Source: CAD feature listing. Evaluate the final solid. Frame: model axes, mm. Face numbers are marked on the shaded views. A direction names the side the tool comes from. Give positions to 0.01 mm unless a question says otherwise; leave off trailing zeros. Order: outer loops, then holes, each group sorted by start corner. A loop starts at its lowest first (then second) coordinate and runs counter-clockwise, first axis right, second up. Notation, with made-up numbers: (54, -5) - (67, -5) arc R18 cw to (67, 19) - close; hole circle Ø6 at (41.25, 1). An arc over 180 degrees is marked (long way). Answer as CSV lines item,"result".
Autodesk Inventor part; units mm, degrees
ref_plane "YZ Plane" through (0, 0, 0) normal (1, 0, 0) x (0, 1, 0)
ref_plane "XZ Plane" through (0, 0, 0) normal (0, 1, 0) x (-1, 0, 0)
ref_plane "XY Plane" through (0, 0, 0) normal (0, 0, 1) x (1, 0, 0)
sketch "Sketch2" plane through (0, 0, 0) normal (0, 1, 0) x (-1, 0, 0)
  circle A0 centre (0, 0) radius 21
  dimension "d1" = 42
extrude "Extrusion1" add sketch "Sketch2" along normal mid plane 16
sketch "Sketch3" plane through (0, -8, 0) normal (0, -1, 0) x (1, 0, 0)
  circle A0 centre (0, 0) radius 21
  dimension "d4" = 42
ref_plane "Work Plane1" through (0, -38, 0) normal (0, -1, 0) x (1, 0, 0)
sketch "Sketch4" plane through (0, -38, 0) normal (0, -1, 0) x (1, 0, 0)
  circle A0 centre (0, 0) radius 28.77
  dimension "d6" = 57.54
loft "Loft1" add profiles "Sketch4" section 1 edges at (21, -8, 0)
sketch "Sketch5" plane through (0, -38, 0) normal (0, -1, 0) x (1, 0, 0)
  circle A0 centre (0, 0) radius 28.77
  line L0 (0, 0) -> (28.77, 0) construction
  line L1 (0, 36.3025) -> (31.4389, 18.1512)
  line L2 (31.4389, 18.1512) -> (31.4389, -18.1512)
  line L3 (31.4389, -18.1512) -> (0, -36.3025)
  line L4 (0, -36.3025) -> (-31.4389, -18.1512)
  line L5 (-31.4389, -18.1512) -> (-31.4389, 18.1512)
  line L6 (-31.4389, 18.1512) -> (0, 36.3025)
ref_plane "Work Plane2" through (0, -68, 0) normal (0, -1, 0) x (1, 0, 0)
sketch "Sketch6" plane through (0, -38, 0) normal (0, -1, 0) x (1, 0, 0)
  point P0 (0, 0)
sketch "Sketch8" plane through (0, -68, 0) normal (0, -1, 0) x (1, 0, 0)
  line L0 (0, 47.0378) -> (40.7359, 23.5189)
  line L1 (40.7359, 23.5189) -> (40.7359, -23.5189)
  line L2 (40.7359, -23.5189) -> (0, -47.0378)
  line L3 (0, -47.0378) -> (-40.7359, -23.5189)
  line L4 (-40.7359, -23.5189) -> (-40.7359, 23.5189)
  line L5 (-40.7359, 23.5189) -> (0, 47.0378)
  point P0 (0, 0)
  point P1 (0, 0)
loft "Loft3" add profiles "Sketch8", "Sketch5" contours all / A0 | L1 L2 L3 L4 L5 L6
sketch "Sketch9" plane through (-40.7359, -68, -23.5189) normal (-0.9551836, 0.296014, 0) x (0, 0, 1)
  line L0 (0, 0) -> (47.0378, 0)
  line L1 (23.5189, 0) -> (16.0189, 0)
  line L2 (31.0189, 0) -> (23.5189, 0)
  line L3 (31.0189, 0) -> (16.0189, 0)
  line L4 (16.0189, 20) -> (31.0189, 20)
  line L5 (23.5189, 0) -> (8.5189, 0)
  line L6 (8.5189, 0) -> (8.5189, 20)
  line L7 (8.5189, 20) -> (38.5189, 20)
  line L8 (38.5189, 20) -> (38.5189, 0)
  point P0 (23.5189, 77.0109)
  dimension "d40" = 15
  dimension "d41" = 20
  dimension "d42" = 30
sketch "Sketch10" plane through (40.7359, -68, 23.5189) normal (0.9551836, 0.296014, 0) x (0, 0, -1)
  line L0 (38.5189, 20) -> (38.5189, 0)
  line L1 (8.5189, 0) -> (8.5189, 20)
  line L2 (8.5189, 20) -> (38.5189, 20)
  line L3 (38.5189, 20) -> (38.5189, 0)
  line L4 (0, 0) -> (47.0378, 0)
  line L5 (8.5189, 0) -> (38.5189, 0)
  point P0 (23.5189, 77.0109)
  point P1 (23.5189, 0)
  point P2 (53.5189, 0)
  point P3 (23.5189, 0)
loft "Loft4" cut profiles "Sketch9", "Sketch10"
ref_plane "Work Plane4" through (0, 63.4475, -18.1512) normal (-1, 0, 0) x (0, 0, 1)
sketch "Sketch12" plane through (0, 63.4475, -18.1512) normal (-1, 0, 0) x (0, 0, 1)
  line L0 (39.1512, -55.4475) -> (-2.8488, -55.4475)
  line L1 (18.1512, -55.4475) -> (39.1512, -55.4475)
  arc A0 (39.1512, -55.4475) -> (50.0417, -31.4475) centre (18.1512, -31.4475) ccw
  line L2 (18.1512, -31.4475) -> (50.0417, -31.4475)
  line L3 (18.1512, -31.4475) -> (18.1512, -55.4475)
  line L4 (18.1512, -55.4475) -> (39.1512, -55.4475)
  point P0 (18.1512, -63.4475)
revolve "Revolution1" add sketch "Sketch12" angle 360 about axis through (0, 32, 0) along (0, -1, 0)
sketch "Sketch14" plane through (0, 63.4475, -18.1512) normal (-1, 0, 0) x (0, 0, 1)
  line L0 (-13.7392, -31.4475) -> (50.0417, -31.4475)
  line L1 (18.1512, -31.4475) -> (33.1512, -31.4475)
  line L2 (18.1512, -31.4475) -> (33.1512, -31.4475) construction
  line L3 (33.1512, -31.4475) -> (33.1512, -45.4475)
  line L4 (33.1512, -45.4475) -> (50.0417, -45.4475)
  line L5 (50.0417, -45.4475) -> (50.0417, -31.4475)
  line L6 (50.0417, -31.4475) -> (33.1512, -31.4475)
  point P0 (18.1512, -63.4475)
  point P1 (33.1512, -31.4475)
  dimension "d47" = 14
  dimension "d48" = 90
  dimension "d49" = 90
extrude "Extrusion2" cut sketch "Sketch14" along normal mid plane 70
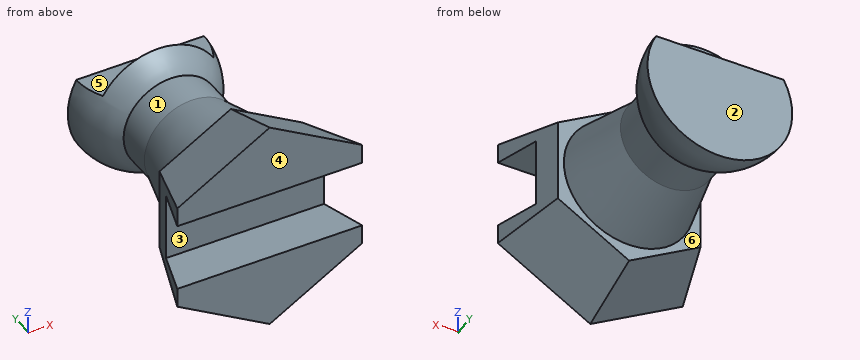
(1) Contact query for flat-ended pins moving along their axis: pin 1 (15.5 mm diameter, centred on x = -2.5, y = 24.5, fed in from +Z); pin 2 (1.5 mm diameter, centred on x = 1.5, y = -17, fed in from -Z); pin 3 (6 mm diameter, centred on x = 4, z = 21, fed in from +Y). Output: stop coordinate, or through.
Completed:
pin 1,"z = 28.65"
pin 2,"z = -23.48"
pin 3,"y = 18"
(2) Cut plane A-A (y = 4.5). Return loops of the section in (x, z), then the cut area to 3 significant figures.
Completed:
outline,"circle Ø42 at (0, 0)"
area,"1,390 mm²"
(3) Ray query, line 1 (Z direction, x = 29, y = -49); line 2 (Z direction, x = 3.5, y = -54.5); line 3 (Y direction, x = -4.5, z = 15.5). Return the intervals inside material, ascending. Write a range as from..to.
Completed:
line 1,"-23.5..-15, 15..23.5"
line 2,"-40.19..-15, 15..40.19"
line 3,"-68..18"
(4) Access query for the marked faces 4, 5 and 6. Directions: +Z, -Z, +X, -X, +Y, -Y. A direction counts if a zero-diameter tool reaches every point of the face in a straight line with its end or side. Return the directions, or none.
Completed:
face 4,"+Z, -Z, +X, -X, -Y"
face 5,"+Z, +X, -X, +Y"
face 6,"none"
(5) Mould query, pull axis Y, two halves, no side actions, for the marked faces 1, 2 and 3. Classes: released by +Y, released by -Y, zero draft, split by the parting line, or undercut.
Completed:
face 1,"undercut"
face 2,"released by +Y"
face 3,"released by -Y"
(6) Cut plane B-B (y = -13.5). Return loops of the section in (x, z).
Completed:
outline,"circle Ø44.85 at (0, 0)"
